```python
from build123d import *

# Parameters (mm, degrees)
F1_DEPTH = 10
F2_W     = 4
F2_H     = 2
F3_DEPTH = 4.5984521023
F4_R     = 0.5


with BuildPart() as f1:
    # F0 (on Right) → F1 (new body, symmetric)
    with BuildSketch(Plane.YZ):
        with BuildLine():
            Line((0, -7.0358098146), (0, 0))
            Line((0, 0), (2, 0))
            Line((2, 0), (2, -4))
            Line((2, -4), (4, -4))
            Line((4, -4), (4, 0))
            Line((4, 0), (4, 4))
            Line((4, 4), (-4, 4))
            Line((-4, 4), (-4, 0))
            Line((-4, 0), (-4, -3.4128310664))
            ThreePointArc((-4, -3.4128310664), (-5.2334442571, -7.0569971371), (-8.4266487834, -9.2028713037))
            Line((-8.4266487834, -9.2028713037), (-22.7866756083, -13.1049798814))
            ThreePointArc((-22.7866756083, -13.1049798814), (-24.3832778714, -14.1779169647), (-25, -16))
            Line((-25, -16), (-25, -21))
            Line((-25, -21), (-25, -23))
            Line((-25, -23), (-20, -23))
            Line((-20, -23), (-20, -21))
            Line((-20, -21), (-22, -21))
            Line((-22, -21), (-22, -16.767326988))
            ThreePointArc((-22, -16.767326988), (-21.7933533403, -16.158565559), (-21.2588190451, -15.8014011617))
            Line((-21.2588190451, -15.8014011617), (-2.9647238196, -10.8995131198))
            ThreePointArc((-2.9647238196, -10.8995131198), (-0.8265866388, -9.4708555306), (0, -7.0358098146))
        make_face()
    extrude(amount=F1_DEPTH, both=True)

    # F2 (on face) → F3 (cut, through all)
    with BuildSketch(Plane(origin=(0, 0, 0), x_dir=(-1, 0, 0), z_dir=(0, 1, 0))):
        with Locations((-5.5, -5.0229031369)):
            Rectangle(F2_W, F2_H)
        with Locations((5.5, -5.0229031369)):
            Rectangle(F2_W, F2_H)
    extrude(amount=-F3_DEPTH, mode=Mode.SUBTRACT)

    # F4
    f4_edges = [f1.edges().sort_by_distance(p)[0] for p in [
        (10, -5.233444, -7.056997),
        (10, -15.606662, -11.153926),
        (10, -22.5, -23),
        (10, -20, -22),
        (10, -21, -21),
        (10, -22, -18.883663),
        (0, -25, -23),
        (-10, -25, -19.5),
        (0, -4, 4),
        (10, 0, 4),
        (10, 1, 0),
        (10, 2, -2),
        (0, 2, -4),
        (10, 3, -4),
        (10, 4, 0),
        (0, 4, 4),
        (-10, 0, 4),
        (-10, -0.826587, -9.470856),
        (-10, 0, -3.517905),
        (-10, 1, 0),
        (-10, 2, -2),
        (-10, 3, -4),
        (-10, 4, 0),
        (-10, -4, 0.293584),
        (-10, -5.233444, -7.056997),
        (-10, -15.606662, -11.153926),
        (-10, -24.383278, -14.177917),
        (-10, -22.5, -23),
        (-10, -20, -22),
        (-10, -21, -21),
        (-10, -22, -18.883663),
        (-10, -21.793353, -16.158566),
        (-10, -12.111771, -13.350457),
        (10, -24.383278, -14.177917),
        (10, -21.793353, -16.158566),
        (0, -20, -21),
        (0, -20, -23),
        (0, 4, -4),
    ]]
    fillet(f4_edges, radius=F4_R)


solid = f1.part
```
Read the model definition and answer for the solid it produces. Units are mm, in the model's axes. A direction names the side the tool comes from. Round coordinates to 2 decimals unless told otherwise and drop trailing zeros. Write each loop counter-clockwise with the first axis right and the second up, starting at its lowest first coordinate (ties: lowest second). Pieces come first, ordered by that corner, then holes. Notation, with made-up numbers: (76.5, 85) - (130.5, 85) arc R31 ccw to (130.5, 119) - close; hole circle Ø5 at (56, 36). An arc over 180 degrees is marked (long way). One line per item, written item: value.
Q1. Find section D-D (z = -17.75). Determine the outline of the cut face in (x, y), and give its area (3 significant figures).
The answers:
outline: (-10, -24.5) arc R0.5 ccw to (-9.5, -25) - (9.5, -25) arc R0.5 ccw to (10, -24.5) - (10, -22.5) arc R0.5 ccw to (9.5, -22) - (-9.5, -22) arc R0.5 ccw to (-10, -22.5) - close
area: 59.8 mm2
Q2. Straight lines are drawn through the part: line 1 (Y direction, x = -9, z = -1.5); line 2 (Y direction, x = 4.25, z = 1.75); line 3 (Y direction, x = -8, z = -21.5). For each, find the intervals that lie inside material, in ascending order. Write a range as from..to.
The answers:
line 1: y = -4..0, 2..4
line 2: y = -4..4
line 3: y = -25..-20
Q3. Find section A-A (z = -3). Determine the outline of the cut face in (x, y), and give its area (3 significant figures).
The answers:
outline: (-10, -3.5) arc R0.5 ccw to (-9.5, -4) - (9.5, -4) arc R0.5 ccw to (10, -3.5) - (10, -0.5) arc R0.5 ccw to (9.5, 0) - (-9.5, 0) arc R0.5 ccw to (-10, -0.5) - close; (-10, 2.5) arc R0.5 ccw to (-9.5, 2) - (9.5, 2) arc R0.5 ccw to (10, 2.5) - (10, 3.5) arc R0.5 ccw to (9.5, 4) - (-9.5, 4) arc R0.5 ccw to (-10, 3.5) - close
area: 120 mm2
Q4. Which of the six approach directions +Z, -Z, +X, -X, +Y, -Y give full straight-line access (tool end or side, diameter ignored) to faces 4 (the flat face through (-5, -2, -6.023)), 5 (the flat face through (0, -4, 0)), 6 (the cylindrical face through (-9.86, -15.67, -11.33)), 7 (the flat face through (-10, -9.5, -10.4)), 8 (the flat face through (0, 0, -4))?
The answers:
face 4: +Y, -Y
face 5: +Z, +X, -X, -Y
face 6: +Z, -X, -Y
face 7: +Z, -Z, -X, +Y, -Y
face 8: -Z, +X, -X
Q5. Each of these flat-tipped pins is pushed along its axis until it touches: P1, Ø1.6, axis at x = -1.5, y = -21, coming from the +Z side; P2, Ø1.5, axis at x = 3.5, z = -6.5, coming from the +Y side; P3, Ø8, axis at x = -6, y = -15.5, coming from the +Z side. Where does it stop, or does it pass through?
The answers:
P1: stops at z = -12.4
P2: stops at y = 0
P3: stops at z = -10.04
Q6. For a pull along Z with two mould halves and no side action, classify faces 1 (the flat face through (0, 1, 0)), 2 (the flat face through (3.5, -2, -5)), 3 (the flat face through (0, 2, -2)) as pulls with the +Z half, pulls with the -Z half, needs draft (parallel to the pull), parting line crosses it, or undercut.
The answers:
face 1: pulls with the -Z half
face 2: undercut
face 3: needs draft
Q7. Find section C-C (x = 8.75). Determine the outline of the cut face in (y, z).
The answers:
outline: (-25, -22.5) arc R0.5 ccw to (-24.5, -23) - (-20.5, -23) arc R0.5 ccw to (-20, -22.5) - (-20, -21.5) arc R0.5 ccw to (-20.5, -21) - (-22, -21) - (-22, -16.77) arc R1 cw to (-21.26, -15.8) - (-2.96, -10.9) arc R4 ccw to (0, -7.04) - (0, 0) - (2, 0) - (2, -3.5) arc R0.5 ccw to (2.5, -4) - (3.5, -4) arc R0.5 ccw to (4, -3.5) - (4, 3.5) arc R0.5 ccw to (3.5, 4) - (-3.5, 4) arc R0.5 ccw to (-4, 3.5) - (-4, -3.41) arc R6 cw to (-8.43, -9.2) - (-22.79, -13.1) arc R3 ccw to (-25, -16) - close
